from build123d import *

# Parameters (mm, degrees)
F0_W     = 863.6
F0_H     = 1022.35
F0_R     = 12.7
F1_DEPTH = 25.4


with BuildPart() as f1:
    # F0 (on Front) → F1 (new body)
    with BuildSketch(Plane.XZ):
        Rectangle(F0_W, F0_H)
        with Locations((-241.3, -422.275)):
            Circle(F0_R, mode=Mode.SUBTRACT)
        with Locations((-292.1, -333.375)):
            Circle(F0_R, mode=Mode.SUBTRACT)
        with Locations((-241.3, -358.775)):
            Circle(F0_R, mode=Mode.SUBTRACT)
        with Locations((-190.5, -422.275)):
            Circle(F0_R, mode=Mode.SUBTRACT)
        with Locations((-190.5, -333.375)):
            Circle(F0_R, mode=Mode.SUBTRACT)
        with Locations((-50.8, -333.375)):
            Circle(F0_R, mode=Mode.SUBTRACT)
        with Locations((-241.3, -168.275)):
            Circle(F0_R, mode=Mode.SUBTRACT)
        with Locations((-292.1, -79.375)):
            Circle(F0_R, mode=Mode.SUBTRACT)
        with Locations((-241.3, -104.775)):
            Circle(F0_R, mode=Mode.SUBTRACT)
        with Locations((-190.5, -168.275)):
            Circle(F0_R, mode=Mode.SUBTRACT)
        with Locations((-190.5, -79.375)):
            Circle(F0_R, mode=Mode.SUBTRACT)
        with Locations((-50.8, -79.375)):
            Circle(F0_R, mode=Mode.SUBTRACT)
        with Locations((0, -422.275)):
            Circle(F0_R, mode=Mode.SUBTRACT)
        with Locations((50.8, -422.275)):
            Circle(F0_R, mode=Mode.SUBTRACT)
        with Locations((0, -358.775)):
            Circle(F0_R, mode=Mode.SUBTRACT)
        with Locations((50.8, -333.375)):
            Circle(F0_R, mode=Mode.SUBTRACT)
        with Locations((190.5, -333.375)):
            Circle(F0_R, mode=Mode.SUBTRACT)
        with Locations((241.3, -422.275)):
            Circle(F0_R, mode=Mode.SUBTRACT)
        with Locations((292.1, -422.275)):
            Circle(F0_R, mode=Mode.SUBTRACT)
        with Locations((241.3, -358.775)):
            Circle(F0_R, mode=Mode.SUBTRACT)
        with Locations((292.1, -333.375)):
            Circle(F0_R, mode=Mode.SUBTRACT)
        with Locations((0, -168.275)):
            Circle(F0_R, mode=Mode.SUBTRACT)
        with Locations((50.8, -168.275)):
            Circle(F0_R, mode=Mode.SUBTRACT)
        with Locations((0, -104.775)):
            Circle(F0_R, mode=Mode.SUBTRACT)
        with Locations((50.8, -79.375)):
            Circle(F0_R, mode=Mode.SUBTRACT)
        with Locations((190.5, -79.375)):
            Circle(F0_R, mode=Mode.SUBTRACT)
        with Locations((241.3, -168.275)):
            Circle(F0_R, mode=Mode.SUBTRACT)
        with Locations((292.1, -168.275)):
            Circle(F0_R, mode=Mode.SUBTRACT)
        with Locations((241.3, -104.775)):
            Circle(F0_R, mode=Mode.SUBTRACT)
        with Locations((292.1, -79.375)):
            Circle(F0_R, mode=Mode.SUBTRACT)
        with Locations((-241.3, 85.725)):
            Circle(F0_R, mode=Mode.SUBTRACT)
        with Locations((-292.1, 174.625)):
            Circle(F0_R, mode=Mode.SUBTRACT)
        with Locations((-241.3, 149.225)):
            Circle(F0_R, mode=Mode.SUBTRACT)
        with Locations((-190.5, 85.725)):
            Circle(F0_R, mode=Mode.SUBTRACT)
        with Locations((-190.5, 174.625)):
            Circle(F0_R, mode=Mode.SUBTRACT)
        with Locations((-50.8, 174.625)):
            Circle(F0_R, mode=Mode.SUBTRACT)
        with Locations((-241.3, 339.725)):
            Circle(F0_R, mode=Mode.SUBTRACT)
        with Locations((-292.1, 428.625)):
            Circle(F0_R, mode=Mode.SUBTRACT)
        with Locations((-241.3, 403.225)):
            Circle(F0_R, mode=Mode.SUBTRACT)
        with Locations((-190.5, 339.725)):
            Circle(F0_R, mode=Mode.SUBTRACT)
        with Locations((-190.5, 428.625)):
            Circle(F0_R, mode=Mode.SUBTRACT)
        with Locations((-50.8, 428.625)):
            Circle(F0_R, mode=Mode.SUBTRACT)
        with Locations((0, 85.725)):
            Circle(F0_R, mode=Mode.SUBTRACT)
        with Locations((50.8, 85.725)):
            Circle(F0_R, mode=Mode.SUBTRACT)
        with Locations((0, 149.225)):
            Circle(F0_R, mode=Mode.SUBTRACT)
        with Locations((50.8, 174.625)):
            Circle(F0_R, mode=Mode.SUBTRACT)
        with Locations((190.5, 174.625)):
            Circle(F0_R, mode=Mode.SUBTRACT)
        with Locations((241.3, 85.725)):
            Circle(F0_R, mode=Mode.SUBTRACT)
        with Locations((292.1, 85.725)):
            Circle(F0_R, mode=Mode.SUBTRACT)
        with Locations((241.3, 149.225)):
            Circle(F0_R, mode=Mode.SUBTRACT)
        with Locations((292.1, 174.625)):
            Circle(F0_R, mode=Mode.SUBTRACT)
        with Locations((0, 339.725)):
            Circle(F0_R, mode=Mode.SUBTRACT)
        with Locations((50.8, 339.725)):
            Circle(F0_R, mode=Mode.SUBTRACT)
        with Locations((0, 403.225)):
            Circle(F0_R, mode=Mode.SUBTRACT)
        with Locations((50.8, 428.625)):
            Circle(F0_R, mode=Mode.SUBTRACT)
        with Locations((190.5, 428.625)):
            Circle(F0_R, mode=Mode.SUBTRACT)
        with Locations((241.3, 339.725)):
            Circle(F0_R, mode=Mode.SUBTRACT)
        with Locations((292.1, 339.725)):
            Circle(F0_R, mode=Mode.SUBTRACT)
        with Locations((241.3, 403.225)):
            Circle(F0_R, mode=Mode.SUBTRACT)
        with Locations((292.1, 428.625)):
            Circle(F0_R, mode=Mode.SUBTRACT)
    extrude(amount=F1_DEPTH)


solid = f1.part
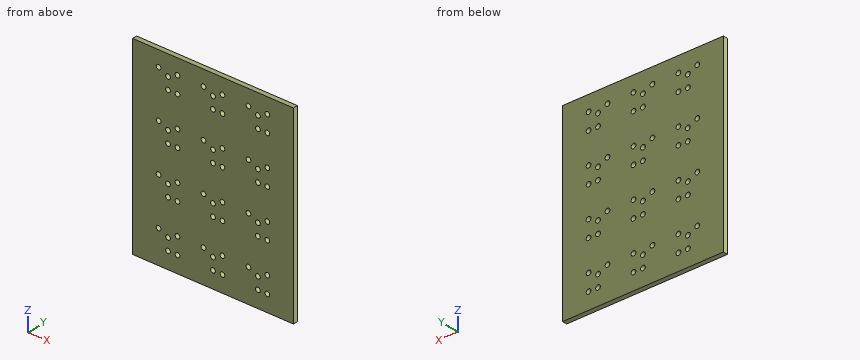
Design review of the part built by this model. Coordinates are the model's own, in mm. Coordinates: 2 decimals unless noted, no trailing zeros. Order: outer loops, then holes, each group sorted by start corner. A loop starts at its lowest first (then second) coordinate and runs counter-clockwise, first axis right, second up. Notation, with made-up numbers: (-2, 7) -> (48, 7) arc R22 cw to (48, 43) -> close; hole circle Ø2 at (38.5, -27). An arc over 180 degrees is marked (long way). One line per item, written item: value.
1) To check wall thickness, follow probe 1 along X at (y, z) = (-23.75, 401); probe 2 along X at (y, z) = (-18.5, -96). State the ranges of each line that lie inside material, in increasing order. Write a range as [from, to].
Output values:
probe 1: x = [-431.8, -253.8], [-228.8, -12.5], [12.5, 228.8], [253.8, 431.8]
probe 2: x = [-431.8, -250.48], [-232.12, -9.18], [9.18, 232.12], [250.48, 431.8]
2) We need section A-A, the plane x = -292.1. Give the boundary of the cut face in (y, z) (3 decimals), then the cut area to 3 significant figures.
Output values:
outline: (-25.4, -511.175) -> (0, -511.175) -> (0, -346.075) -> (-25.4, -346.075) -> close; (-25.4, -320.675) -> (0, -320.675) -> (0, -92.075) -> (-25.4, -92.075) -> close; (-25.4, -66.675) -> (0, -66.675) -> (0, 161.925) -> (-25.4, 161.925) -> close; (-25.4, 187.325) -> (0, 187.325) -> (0, 415.925) -> (-25.4, 415.925) -> close; (-25.4, 441.325) -> (0, 441.325) -> (0, 511.175) -> (-25.4, 511.175) -> close
area: 23,400 mm2
3) Clearance check with a flat-ended pin moving along its axis: P1, Ø15, axis at x = 241.3, z = -422.275, coming from the -Y side. State where the tip first meets the part, or that it passes through.
Output values:
P1: passes through
4) We need section B-B, the plane x = 50.8. Count the separate pieces of the cut face and the enclosed holes in it, then the cut area to 3 significant figures.
Output values:
separate pieces: 9
enclosed holes: 0
area: 20,800 mm2
